```python
from build123d import *

# Parameters (mm, degrees)
F0_W      = 30
F0_H      = 20
F1_DEPTH  = 15
F2_W      = 5
F2_H      = 15
F3_DEPTH  = 25
F4_W      = 5
F4_H      = 15
F5_DEPTH  = 25
F6_R      = 5
F7_DEPTH  = 15.001
F8_R      = 2
F10_R     = 1
F11_DEPTH = 25
F9_R      = 1
F12_DEPTH = 5.001


with BuildPart() as f1:
    # F0 (on Top) → F1 (new body)
    with BuildSketch(Plane.XY):
        with Locations((3.173804, 4.413379)):
            Rectangle(F0_W, F0_H)
    extrude(amount=F1_DEPTH)

    # F2 (on face) → F3 (cut)
    with BuildSketch(Plane.XY.offset(15)):
        with Locations((15.673804, 6.913379)):
            Rectangle(F2_W, F2_H)
    extrude(amount=-F3_DEPTH, mode=Mode.SUBTRACT)

    # F4 (on face) → F5 (cut)
    with BuildSketch(Plane.XY.offset(15)):
        with Locations((-9.326196, 6.913379)):
            Rectangle(F4_W, F4_H)
    extrude(amount=-F5_DEPTH, mode=Mode.SUBTRACT)

    # F6 (on face) → F7 (cut, through all)
    with BuildSketch(Plane.XY.offset(15)):
        with Locations((3.173804, 6.913379)):
            Circle(F6_R)
    extrude(amount=-F7_DEPTH, mode=Mode.SUBTRACT)

    # F8
    f8_edges = [f1.edges().sort_by_distance(p)[0] for p in [
        (-6.826196, -0.586621, 7.5),
        (13.173804, -0.586621, 7.5),
    ]]
    fillet(f8_edges, radius=F8_R)

    # F10 (on face) → F11 (cut)
    with BuildSketch(Plane(origin=(0, -0.586621, 0), x_dir=(-1, 0, 0), z_dir=(0, 1, 0))):
        with Locations((10.326196, 7.5)):
            Circle(F10_R)
    extrude(amount=-F11_DEPTH, mode=Mode.SUBTRACT)

    # F9 (on face) → F12 (cut, through all)
    with BuildSketch(Plane(origin=(0, -0.586621, 0), x_dir=(-1, 0, 0), z_dir=(0, 1, 0))):
        with Locations((-16.673804, 7.5)):
            Circle(F9_R)
    extrude(amount=-F12_DEPTH, mode=Mode.SUBTRACT)


solid = f1.part
```
Work out the finished part from the listing and answer in its coordinate system (mm). A direction names the side the tool comes from. Round coordinates to 2 decimals unless told otherwise and drop trailing zeros. Write each loop counter-clockwise with the first axis right and the second up, starting at its lowest first coordinate (ties: lowest second). Pieces come first, ordered by that corner, then holes.
1) Determine the mould class of faces 1 (the face through (-9.589, -3.052, 8.176)), 2 (the face through (6, 2, 15)), 3 (the face through (5.481, 2.478, 7.605)) for opening direction Z: pulls with the +Z half, pulls with the -Z half, needs draft (parallel to the pull), parting line crosses it, or undercut.
2) A cutting plane is placed at D-D on z = 12. Determine the outline of the cut face in (x, y), and give its area (3 significant figures).
3) Flat-ended cylindrical pins translate along their axes: P1, Ø3.5, axis at x = 17.5, z = 10, coming from the +Y side; P2, Ø4, axis at y = 9.5, z = 8, coming from the +X side; P3, Ø4, axis at y = 7, z = 6.5, coming from the -X side. Find the tip coordinate at first contact, or state that the pin passes through.
4) Consider probe 1 along Z at (x, y) = (16.75, -3.75); probe 2 along Y at (x, z) = (15.25, 2.5); probe 3 along Y at (x, z) = (5.5, 5.25). Determine where each line is inside the solid, lowest interval first.
5) A cutting plane is placed at B-B on y = 3.25. Determine the outline of the cut face in (x, z).
6) Which of the six approach directions +Z, -Z, +X, -X, +Y, -Y give full straight-line access (tool end or side, diameter ignored) to faces 4 (the face through (13.174, 8, 8)), 5 (the face through (15.72, -3.05, 7.8)), 6 (the face through (-9, -0.587, 8))?
7) A cutting plane is placed at C-C on x = -9.75. Determine the outline of the cut face in (y, z), and give its area (3 significant figures).
8) A cutting plane is placed at A-A on z = 7.5. Determine the outline of the cut face in (x, y).
Entries:
1. face 1: undercut
1. face 2: pulls with the +Z half
1. face 3: needs draft
2. outline: (-11.83, -5.59) - (18.17, -5.59) - (18.17, -0.59) - (15.17, -0.59) arc R2 cw to (13.17, 1.41) - (13.17, 14.41) - (-6.83, 14.41) - (-6.83, 1.41) arc R2 cw to (-8.83, -0.59) - (-11.83, -0.59) - close; hole circle Ø10 at (3.17, 6.91)
2. area: 373 mm2
3. P1: stops at y = -0.59
3. P2: stops at x = 13.17
3. P3: stops at x = -6.83
4. probe 1: z = 0 to 6.5, 8.5 to 15
4. probe 2: y = -5.59 to -0.59
4. probe 3: y = -5.59 to 2.49, 11.34 to 14.41
5. outline: (-6.83, 0) - (-0.23, 0) - (-0.23, 15) - (-6.83, 15) - close; (6.58, 0) - (13.17, 0) - (13.17, 15) - (6.58, 15) - close
6. face 4: +Z, -Z, +X, +Y
6. face 5: +Y, -Y
6. face 6: +Z, -Z, -X, +Y
7. outline: (-5.59, 0) - (-0.59, 0) - (-0.59, 6.68) - (-5.59, 6.68) - close; (-5.59, 8.32) - (-0.59, 8.32) - (-0.59, 15) - (-5.59, 15) - close
7. area: 66.8 mm2
8. outline: (-11.83, -5.59) - (-11.33, -5.59) - (-11.33, -0.59) - (-11.83, -0.59) - close; (-9.33, -5.59) - (15.67, -5.59) - (15.67, -0.59) - (15.17, -0.59) arc R2 cw to (13.17, 1.41) - (13.17, 14.41) - (-6.83, 14.41) - (-6.83, 1.41) arc R2 cw to (-8.83, -0.59) - (-9.33, -0.59) - close; (17.67, -5.59) - (18.17, -5.59) - (18.17, -0.59) - (17.67, -0.59) - close; hole circle Ø10 at (3.17, 6.91)
